Geometry: final body of the model. Coordinates: model frame, mm. Round coordinates to 2 decimals unless told otherwise and drop trailing zeros. Write each loop counter-clockwise with the first axis right and the second up, starting at its lowest first coordinate (ties: lowest second). Pieces come first, ordered by that corner, then holes.
from build123d import *

# Parameters (mm, degrees)
PLACA_START                    = 46.75
SK_PLACA_W                     = 70
SK_PLACA_H                     = 160
PLACA_DEPTH                    = 6.35
EXTREMOS_START                 = 46.75
SK_EXTREMOS_R                  = 35
EXTREMOS_DEPTH                 = 6.35
PASANTES_M4_SEPARADORES_START  = 46.75
SK_PASANTES_M4_SEPARADORES_R   = 2.25
PASANTES_M4_SEPARADORES_DEPTH  = 6.35
ASIENTO_J3_START               = 38.75
SK_ASIENTO_J3_R                = 30
SK_ASIENTO_J3_R_2              = 17.5
ASIENTO_J3_DEPTH               = 8
PASO_ROTOR_J3_START            = 38.75
SK_PASO_ROTOR_J3_R             = 17.5
PASO_ROTOR_J3_DEPTH            = 14.35
PASANTES_M2_5_ESTATOR_J3_START = 38.75
SK_PASANTES_M2_5_ESTATOR_J3_R  = 1.45
PASANTES_M2_5_ESTATOR_J3_DEPTH = 14.35
CAJAS_M2_5_J3_START            = 50.6
SK_CAJAS_M2_5_J3_R             = 2.75
CAJAS_M2_5_J3_DEPTH            = 2.5
PASANTES_M4_SALIDA_J2_START    = 46.75
SK_PASANTES_M4_SALIDA_J2_R     = 2.25
PASANTES_M4_SALIDA_J2_DEPTH    = 6.35
CAJAS_M4_J2_START              = 49.6
SK_CAJAS_M4_J2_R               = 4
CAJAS_M4_J2_DEPTH              = 3.5
PASANTE_M3_CINCHO_START        = 46.75
SK_PASANTE_M3_CINCHO_R         = 1.7
PASANTE_M3_CINCHO_DEPTH        = 6.35
SK_CAJAS_M4_SEPARADORES_R      = 4
CAJAS_M4_SEPARADORES_DEPTH     = 3.5


with BuildPart() as part:
    # Sk_Placa → Placa (new body)
    with BuildSketch(Plane(origin=(0, 0, 0), x_dir=(1, 0, 0), z_dir=(0, 1, 0)).offset(PLACA_START)):
        with Locations((0, -250)):
            Rectangle(SK_PLACA_W, SK_PLACA_H)
    extrude(amount=PLACA_DEPTH)

    # Sk_Extremos → Extremos (add)
    with BuildSketch(Plane(origin=(0, 0, 0), x_dir=(1, 0, 0), z_dir=(0, 1, 0)).offset(EXTREMOS_START)):
        with Locations((0, -170)):
            Circle(SK_EXTREMOS_R)
        with Locations((0, -330)):
            Circle(SK_EXTREMOS_R)
    extrude(amount=EXTREMOS_DEPTH)

    # Sk_Pasantes_M4_separadores → Pasantes_M4_separadores (cut)
    with BuildSketch(Plane(origin=(0, 0, 0), x_dir=(1, 0, 0), z_dir=(0, 1, 0)).offset(PASANTES_M4_SEPARADORES_START)):
        with Locations(Location((0, -250, 0), (0, 0, 270))):
            Circle(SK_PASANTES_M4_SEPARADORES_R)
        with Locations(Location((-22, -300, 0), (0, 0, 270))):
            Circle(SK_PASANTES_M4_SEPARADORES_R)
        with Locations(Location((22, -300, 0), (0, 0, 270))):
            Circle(SK_PASANTES_M4_SEPARADORES_R)
    extrude(amount=PASANTES_M4_SEPARADORES_DEPTH, mode=Mode.SUBTRACT)

    # Sk_Asiento_J3 → Asiento_J3 (add)
    with BuildSketch(Plane(origin=(0, 0, 0), x_dir=(1, 0, 0), z_dir=(0, 1, 0)).offset(ASIENTO_J3_START)):
        with Locations(Location((0, -330, 0), (0, 0, 270))):
            Circle(SK_ASIENTO_J3_R)
        with Locations(Location((0, -330, 0), (0, 0, 270))):
            Circle(SK_ASIENTO_J3_R_2, mode=Mode.SUBTRACT)
    extrude(amount=ASIENTO_J3_DEPTH)

    # Sk_Paso_rotor_J3 → Paso_rotor_J3 (cut)
    with BuildSketch(Plane(origin=(0, 0, 0), x_dir=(1, 0, 0), z_dir=(0, 1, 0)).offset(PASO_ROTOR_J3_START)):
        with Locations(Location((0, -330, 0), (0, 0, 270))):
            Circle(SK_PASO_ROTOR_J3_R)
    extrude(amount=PASO_ROTOR_J3_DEPTH, mode=Mode.SUBTRACT)

    # Sk_Pasantes_M2-5_estator_J3 → Pasantes_M2-5_estator_J3 (cut)
    with BuildSketch(Plane(origin=(0, 0, 0), x_dir=(1, 0, 0), z_dir=(0, 1, 0)).offset(PASANTES_M2_5_ESTATOR_J3_START)):
        with Locations(Location((20.289983175, -329.362361591, 0), (0, 0, 270))):
            Circle(SK_PASANTES_M2_5_ESTATOR_J3_R)
        with Locations(Location((14.798063137, -343.89630625, 0), (0, 0, 270))):
            Circle(SK_PASANTES_M2_5_ESTATOR_J3_R)
        with Locations(Location((0.637638409, -350.289983175, 0), (0, 0, 270))):
            Circle(SK_PASANTES_M2_5_ESTATOR_J3_R)
        with Locations(Location((-13.89630625, -344.798063137, 0), (0, 0, 270))):
            Circle(SK_PASANTES_M2_5_ESTATOR_J3_R)
        with Locations(Location((-20.289983175, -330.637638409, 0), (0, 0, 270))):
            Circle(SK_PASANTES_M2_5_ESTATOR_J3_R)
        with Locations(Location((-14.798063137, -316.10369375, 0), (0, 0, 270))):
            Circle(SK_PASANTES_M2_5_ESTATOR_J3_R)
        with Locations(Location((-0.637638409, -309.710016825, 0), (0, 0, 270))):
            Circle(SK_PASANTES_M2_5_ESTATOR_J3_R)
        with Locations(Location((13.89630625, -315.201936863, 0), (0, 0, 270))):
            Circle(SK_PASANTES_M2_5_ESTATOR_J3_R)
    extrude(amount=PASANTES_M2_5_ESTATOR_J3_DEPTH, mode=Mode.SUBTRACT)

    # Sk_Cajas_M2-5_J3 → Cajas_M2-5_J3 (cut)
    with BuildSketch(Plane(origin=(0, 0, 0), x_dir=(1, 0, 0), z_dir=(0, 1, 0)).offset(CAJAS_M2_5_J3_START)):
        with Locations(Location((20.289983175, -329.362361591, 0), (0, 0, 270))):
            Circle(SK_CAJAS_M2_5_J3_R)
        with Locations(Location((14.798063137, -343.89630625, 0), (0, 0, 270))):
            Circle(SK_CAJAS_M2_5_J3_R)
        with Locations(Location((0.637638409, -350.289983175, 0), (0, 0, 270))):
            Circle(SK_CAJAS_M2_5_J3_R)
        with Locations(Location((-13.89630625, -344.798063137, 0), (0, 0, 270))):
            Circle(SK_CAJAS_M2_5_J3_R)
        with Locations(Location((-20.289983175, -330.637638409, 0), (0, 0, 270))):
            Circle(SK_CAJAS_M2_5_J3_R)
        with Locations(Location((-14.798063137, -316.10369375, 0), (0, 0, 270))):
            Circle(SK_CAJAS_M2_5_J3_R)
        with Locations(Location((-0.637638409, -309.710016825, 0), (0, 0, 270))):
            Circle(SK_CAJAS_M2_5_J3_R)
        with Locations(Location((13.89630625, -315.201936863, 0), (0, 0, 270))):
            Circle(SK_CAJAS_M2_5_J3_R)
    extrude(amount=CAJAS_M2_5_J3_DEPTH, mode=Mode.SUBTRACT)

    # Sk_Pasantes_M4_salida_J2 → Pasantes_M4_salida_J2 (cut)
    with BuildSketch(Plane(origin=(0, 0, 0), x_dir=(1, 0, 0), z_dir=(0, 1, 0)).offset(PASANTES_M4_SALIDA_J2_START)):
        with Locations(Location((14.839084994, -167.808754572, 0), (0, 0, 270))):
            Circle(SK_PASANTES_M4_SALIDA_J2_R)
        with Locations(Location((9.317216704, -181.75540186, 0), (0, 0, 270))):
            Circle(SK_PASANTES_M4_SALIDA_J2_R)
        with Locations(Location((-5.52186829, -183.946647288, 0), (0, 0, 270))):
            Circle(SK_PASANTES_M4_SALIDA_J2_R)
        with Locations(Location((-14.839084994, -172.191245428, 0), (0, 0, 270))):
            Circle(SK_PASANTES_M4_SALIDA_J2_R)
        with Locations(Location((-9.317216704, -158.24459814, 0), (0, 0, 270))):
            Circle(SK_PASANTES_M4_SALIDA_J2_R)
        with Locations(Location((5.52186829, -156.053352712, 0), (0, 0, 270))):
            Circle(SK_PASANTES_M4_SALIDA_J2_R)
    extrude(amount=PASANTES_M4_SALIDA_J2_DEPTH, mode=Mode.SUBTRACT)

    # Sk_Cajas_M4_J2 → Cajas_M4_J2 (cut)
    with BuildSketch(Plane(origin=(0, 0, 0), x_dir=(1, 0, 0), z_dir=(0, 1, 0)).offset(CAJAS_M4_J2_START)):
        with Locations(Location((14.839084994, -167.808754572, 0), (0, 0, 270))):
            Circle(SK_CAJAS_M4_J2_R)
        with Locations(Location((9.317216704, -181.75540186, 0), (0, 0, 270))):
            Circle(SK_CAJAS_M4_J2_R)
        with Locations(Location((-5.52186829, -183.946647288, 0), (0, 0, 270))):
            Circle(SK_CAJAS_M4_J2_R)
        with Locations(Location((-14.839084994, -172.191245428, 0), (0, 0, 270))):
            Circle(SK_CAJAS_M4_J2_R)
        with Locations(Location((-9.317216704, -158.24459814, 0), (0, 0, 270))):
            Circle(SK_CAJAS_M4_J2_R)
        with Locations(Location((5.52186829, -156.053352712, 0), (0, 0, 270))):
            Circle(SK_CAJAS_M4_J2_R)
    extrude(amount=CAJAS_M4_J2_DEPTH, mode=Mode.SUBTRACT)

    # Sk_Pasante_M3_cincho → Pasante_M3_cincho (cut)
    with BuildSketch(Plane(origin=(0, 0, 0), x_dir=(1, 0, 0), z_dir=(0, 1, 0)).offset(PASANTE_M3_CINCHO_START)):
        with Locations(Location((-22, -230, 0), (0, 0, 270))):
            Circle(SK_PASANTE_M3_CINCHO_R)
    extrude(amount=PASANTE_M3_CINCHO_DEPTH, mode=Mode.SUBTRACT)

    # Sk_Cajas_M4_separadores → Cajas_M4_separadores (cut)
    with BuildSketch(Plane(origin=(0, 53.1, 0), x_dir=(1, 0, 0), z_dir=(0, 1, 0))):
        with Locations(Location((0, -250, 0), (0, 0, 270))):
            Circle(SK_CAJAS_M4_SEPARADORES_R)
        with Locations(Location((22, -300, 0), (0, 0, 270))):
            Circle(SK_CAJAS_M4_SEPARADORES_R)
        with Locations(Location((-22, -300, 0), (0, 0, 270))):
            Circle(SK_CAJAS_M4_SEPARADORES_R)
    extrude(amount=-CAJAS_M4_SEPARADORES_DEPTH, mode=Mode.SUBTRACT)


solid = part.part
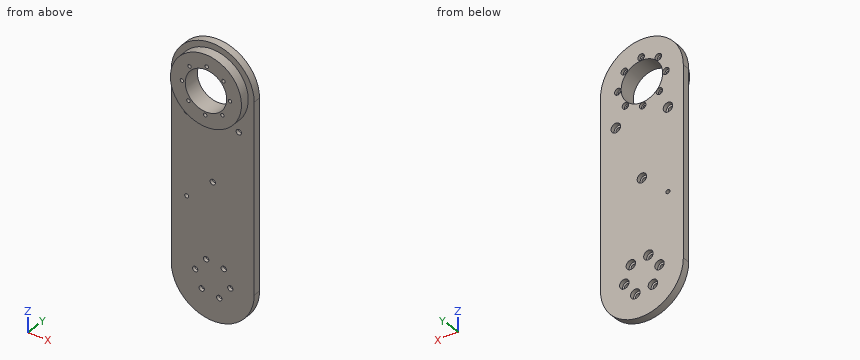
1) Section B-B on y = 44.25. State how many separate pieces and enclosed holes the cut face has, plus the area to 3 significant figures.
2) First-contact query: P1, Ø2, axis at x = -10.5, y = 40.5, coming from the +Z side; P2, Ø6, axis at y = 45.5, z = 233, coming from the -X side; P3, Ø10.5, axis at x = -9.32, z = 158.24, coming from the -Y side; P4, Ø6.5, axis at x = 14.5, z = 168, coming from the +Y side. Flat tips, straight axial feed; report the tip coordinate or a pass-through.
3) Section A-A on z = 250. Output: boundary loops of the cut face in (x, y), plus the area to 3 significant figures.
4) Line query: probe 1 along Z at (x, y) = (-1, 43.75); probe 2 along Z at (x, y) = (-20, 48.5); probe 3 along Z at (x, y) = (-3.5, 45.75). Output: solid intervals per line, ascending.
5) Section C-C on z = 200.5. Output: boundary loops of the cut face in (x, y).
Filled in:
1. separate pieces: 1
1. enclosed holes: 9
1. area: 1,810 mm2
2. P1: stops at z = 358.46
2. P2: stops at x = -35
2. P3: stops at y = 46.75
2. P4: stops at y = 49.6
3. outline: (-35, 46.75) - (-2.25, 46.75) - (-2.25, 49.6) - (-4, 49.6) - (-4, 53.1) - (-35, 53.1) - close; (2.25, 46.75) - (35, 46.75) - (35, 53.1) - (4, 53.1) - (4, 49.6) - (2.25, 49.6) - close
3. area: 404 mm2
4. probe 1: z = 300.02 to 308.31, 311.11 to 312.53, 347.47 to 359.98
4. probe 2: z = 141.28 to 298.97, 301.03 to 329.22, 332.06 to 358.72
4. probe 3: z = 300.2 to 312.85, 347.15 to 359.8
5. outline: (-35, 46.75) - (35, 46.75) - (35, 53.1) - (-35, 53.1) - close
